```python
from build123d import *

# Parameters (mm, degrees)
SKETCH316_R      = 1
EXTRUDE183_DEPTH = 9.4
SKETCH317_R      = 2
EXTRUDE184_DEPTH = 9.4


with BuildPart() as extrude183:
    # Sketch316 → Extrude183 (new body)
    with BuildSketch(Plane.XY.offset(6.6)):
        with Locations((36, -22)):
            Circle(SKETCH316_R)
    extrude(amount=EXTRUDE183_DEPTH)


with BuildPart() as cut082:
    # Sketch317 → Extrude184 (new body)
    with BuildSketch(Plane.XY.offset(6.6)):
        with Locations((36, -22)):
            Circle(SKETCH317_R)
    extrude(amount=EXTRUDE184_DEPTH)

    # Cut082: cut Extrude183
    add(extrude183.part, mode=Mode.SUBTRACT)


with BuildPart() as cut082_1:
    # Cut082 placement: moved
    add(cut082.part.moved(Location((-51, 44, 0))))


solid = cut082_1.part
```
The model under review builds one solid part; all positions refer to its coordinate system, in mm. Round coordinates to 2 decimals unless told otherwise and drop trailing zeros. Write each loop counter-clockwise with the first axis right and the second up, starting at its lowest first coordinate (ties: lowest second). Pieces come first, ordered by that corner, then holes. Notation, with made-up numbers: (77.5, 78) -> (121.5, 78) arc R25 ccw to (121.5, 91) -> close; hole circle Ø7 at (31.25, 56.5). An arc over 180 degrees is marked (long way). Use CSV: the item, a comma, the result in double quotes.
Q1. Mouldability with a two-part tool opening along Y and no side actions: class faces 1 (the cylindrical face through (-17, 22, 11)), 2 (the flat face through (-14, 21, 16)), 3 (the cylindrical face through (-15, 21, 11)) as released by +Y, released by -Y, zero draft, split by the parting line, or undercut.
Checks:
face 1,"split by the parting line"
face 2,"zero draft"
face 3,"undercut"
Q2. Consider section C-C (z = 8). Give the boundary of the cut face in (x, y).
Checks:
outline,"circle Ø4 at (-15, 22); hole circle Ø2 at (-15, 22)"
Q3. To check wall thickness, follow probe 1 along Y at (x, z) = (-15, 9.5); probe 2 along X at (y, z) = (22.3, 10.5); probe 3 along Y at (x, z) = (-15.55, 9.25). State the ranges of each line that lie inside material, in increasing order. Write a range as [from, to].
Checks:
probe 1,"[20, 21], [23, 24]"
probe 2,"[-16.98, -15.95], [-14.05, -13.02]"
probe 3,"[20.08, 21.16], [22.84, 23.92]"
Q4. Consider section D-D (x = -13.45). Give the boundary of the cut face in (y, z), then the cut area to 3 significant figures.
Checks:
outline,"(20.74, 6.6) -> (23.26, 6.6) -> (23.26, 16) -> (20.74, 16) -> close"
area,"23.8 mm²"
Q5. Consider section B-B (y = 22). Give the boundary of the cut face in (x, z), then the cut area to 3 significant figures.
Checks:
outline,"(-17, 6.6) -> (-16, 6.6) -> (-16, 16) -> (-17, 16) -> close; (-14, 6.6) -> (-13, 6.6) -> (-13, 16) -> (-14, 16) -> close"
area,"18.8 mm²"
Q6. Consider section A-A (x = -15). Give the boundary of the cut face in (y, z), then the cut area to 3 significant figures.
Checks:
outline,"(20, 6.6) -> (21, 6.6) -> (21, 16) -> (20, 16) -> close; (23, 6.6) -> (24, 6.6) -> (24, 16) -> (23, 16) -> close"
area,"18.8 mm²"
